Design review of the part shown in the three views and the two pictorial views. Dimensions are in mm from the part's minimum x, y and z. A direction names the side the tool comes from. Give positions to 0.01 mm unless a question says otherwise; leave off trailing zeros. Loops run counter-clockwise (first coordinate to the right, second up) from the corner with the lowest first, then second, coordinate; pieces in that order, holes last. Notation, with made-up numbers: (38.25, 50) -> (69.25, 50) arc R28 cw to (69.25, 81) -> close; hole circle Ø8 at (10, 35.25). An arc over 180 degrees is marked (long way). Answer as CSV lines item,"result".
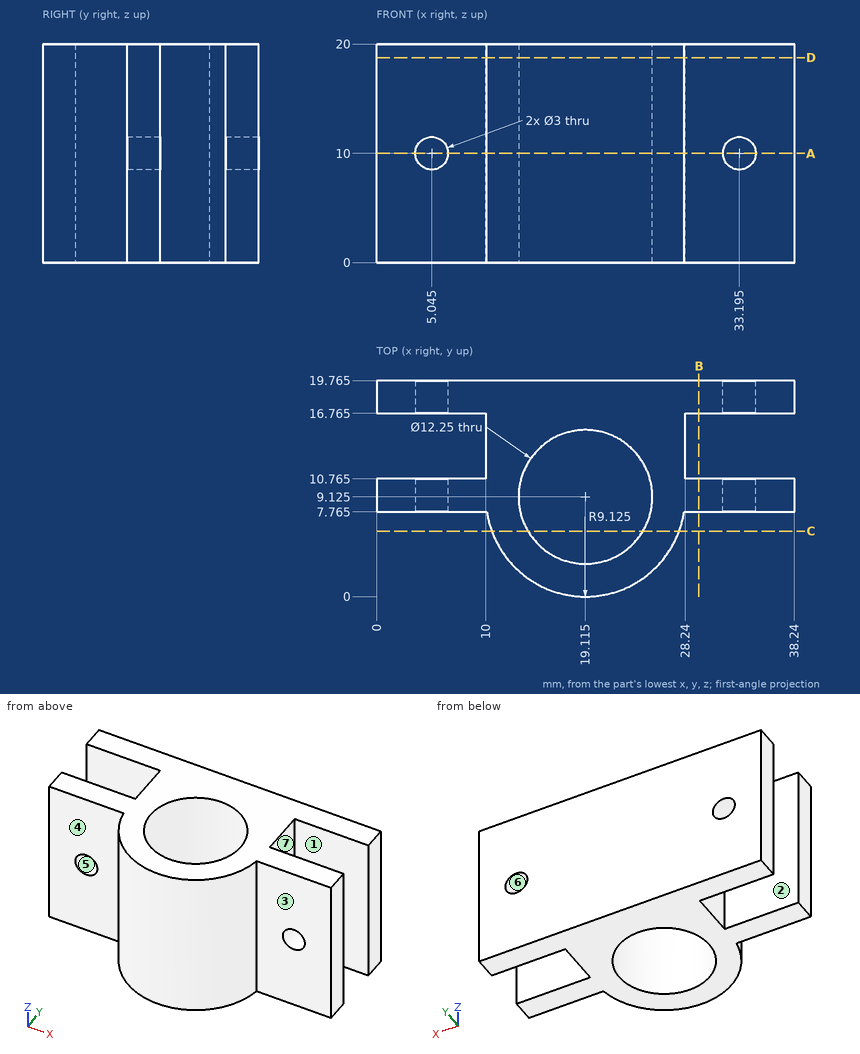
Q1. The part is to be moulded in two halves that separate along X. For the marked faces 4, 5, 6 and 7, say which applies: pulls with the +X half, pulls with the -X half, needs draft (parallel to the pull), parting line crosses it, or undercut.
Filled sheet:
face 4,"needs draft"
face 5,"undercut"
face 6,"undercut"
face 7,"pulls with the +X half"
Q2. To check wall thickness, follow probe 1 along Y at (x, z) = (36, 13.75) (3 decimals); probe 2 along Y at (x, z) = (23, 17) (1 decimal); probe 3 along X at (y, z) = (11.5, 2). State the ranges of each line that lie inside material, in increasing order. Write a range as from..to.
Filled sheet:
probe 1,"y = 7.765..10.765, 16.765..19.765"
probe 2,"y = 0.9..4.4, 13.9..19.8"
probe 3,"x = 10..13.47, 24.76..28.24"
Q3. We need section C-C, the plane y = 6. State the section outline as (x, z) points, and give its area (3 significant figures).
Filled sheet:
outline,"(10.54, 0) -> (13.85, 0) -> (13.85, 20) -> (10.54, 20) -> close; (24.38, 0) -> (27.69, 0) -> (27.69, 20) -> (24.38, 20) -> close"
area,"132 mm^2"
Q4. Clearance check with flat-ended pins moving along their axes: pin 1 Ø3 at (y, z) = (13, 11.5) entering from -X; pin 2 Ø7.5 at (x, y) = (19.12, 9.12) entering from +Z; pin 3 Ø8 at (x, z) = (31, 12) entering from -Y; pin 4 Ø8 at (y, z) = (2.5, 4) entering from -X. State where each tip first meets the part, or that it passes through.
Filled sheet:
pin 1,"stops at x = 10"
pin 2,"passes through"
pin 3,"stops at y = 4.53"
pin 4,"stops at x = 10.38"
Q5. We need section D-D, the plane z = 18.75. State the section outline as (x, y) points (3 decimals), and give its area (3 significant figures).
Filled sheet:
outline,"(0, 7.765) -> (10.092, 7.765) arc R9.125 ccw to (28.138, 7.765) -> (38.24, 7.765) -> (38.24, 10.765) -> (28.24, 10.765) -> (28.24, 16.765) -> (38.24, 16.765) -> (38.24, 19.765) -> (0, 19.765) -> (0, 16.765) -> (10, 16.765) -> (10, 10.765) -> (0, 10.765) -> close; hole circle Ø12.25 at (19.115, 9.125)"
area,"327 mm^2"
Q6. We need section A-A, the plane z = 10. State how many separate pieces and enclosed holes the cut face has, and give its area (3 significant figures).
Filled sheet:
separate pieces,"5"
enclosed holes,"1"
area,"291 mm^2"
Q7. We need section B-B, the plane x = 29.5. State the section outline as (y, z) points (3 decimals), and give its area (3 significant figures).
Filled sheet:
outline,"(7.765, 0) -> (10.765, 0) -> (10.765, 20) -> (7.765, 20) -> close; (16.765, 0) -> (19.765, 0) -> (19.765, 20) -> (16.765, 20) -> close"
area,"120 mm^2"
Q8. For the marked faces 1, 2 and 3, list the 3-axis set-ups (+Z, -Z, +X, -X, +Y, -Y) from which the entire face can be reached by the end or side of a thin tool; tool diameter is ignored.
Filled sheet:
face 1,"+Z, -Z, +X"
face 2,"+Z, -Z, -X"
face 3,"+Z, -Z, +X, -Y"
